Input: part model. Units: mm. Frame: model coordinates. Face numbers are marked on the shaded views. A direction names the side the tool comes from. Give positions to 0.01 mm unless a question says otherwise; leave off trailing zeros. Order: outer loops, then holes, each group sorted by start corner. A loop starts at its lowest first (then second) coordinate and runs counter-clockwise, first axis right, second up. Notation, with made-up numbers: (84.25, 43) - (95.25, 43) arc R12 cw to (95.25, 53) - close; hole circle Ø10 at (-8.75, 35). An arc over 180 degrees is marked (long way). Use a Markdown table: item, result.
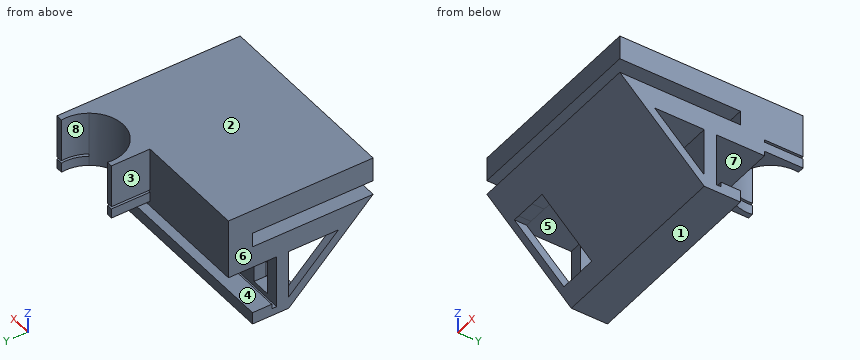
Autodesk Inventor part; units mm, degrees
ref_plane "YZ Plane" through (0, 0, 0) normal (1, 0, 0) x (0, 1, 0)
ref_plane "XZ Plane" through (0, 0, 0) normal (0, 1, 0) x (-1, 0, 0)
ref_plane "XY Plane" through (0, 0, 0) normal (0, 0, 1) x (1, 0, 0)
sketch "Base" plane through (0, 0, 0) normal (1, 0, 0) x (0, 1, 0)
  line L0 (0, 0) -> (0, 6)
  line L1 (0, 6) -> (-50, 6)
  line L2 (-50, 6) -> (-50, 16)
  line L3 (-50, 16) -> (10, 16)
  line L4 (10, -9) -> (-10, -9)
  line L5 (-10, -9) -> (-10, -29)
  line L6 (-10, -29) -> (0, -29)
  line L7 (0, -29) -> (0, -34)
  line L8 (0, -34) -> (-15, -34)
  line L9 (-15, -34) -> (-50, 0)
  line L10 (-50, 0) -> (0, 0)
  line L11 (10, 16) -> (10, -9)
  dimension "d0" = 6
  dimension "d1" = 50
  dimension "d2" = 10
  dimension "d3" = 60
  dimension "d4" = 25
  dimension "d5" = 20
  dimension "d6" = 20
  dimension "d7" = 10
  dimension "d8" = 5
  dimension "d9" = 15
sketch "Mount" plane through (0, 0, 0) normal (1, 0, 0) x (0, 1, 0)
  line L0 (10, 16) -> (26, 16)
  line L1 (26, 16) -> (26, -7)
  line L2 (26, -7) -> (10, -7)
  line L3 (10, -7) -> (10, 16)
  point P0 (0, 0)
  dimension "d13" = 16
  dimension "d14" = 23
extrude "Extrusion1" add sketch "Base" along normal blind 90
extrude "Extrusion2" add sketch "Mount" along normal blind 90
sketch "Sketch4" plane through (0, 10, -7) normal (0, 0, -1) x (-1, 0, 0)
  line L0 (0, 0) -> (0, 16)
  line L1 (0, 16) -> (-90, 16)
  line L2 (-90, 0) -> (-90, 16)
  line L3 (0, 0) -> (-90, 0)
  line L4 (-90, 17.3769) -> (-85, 17.3769)
  line L5 (-85, 17.3769) -> (-85, 0)
  line L6 (0, 0) -> (-90, 0)
  line L7 (-85, 0) -> (-62.2, 0)
  line L8 (-62.2, 0) -> (-62.2, 17.3769)
  line L9 (-62.2, 17.3769) -> (-57.2, 17.3769)
  line L10 (-57.2, 17.3769) -> (-57.2, 0)
  line L11 (-90, 17.3769) -> (-90, 25.7938)
  line L12 (-90, 25.7938) -> (16.0885, 26.6461)
  line L13 (16.0885, 26.6461) -> (17.0474, 0)
  line L14 (17.0474, 0) -> (-57.2, 0)
  point P0 (0, -10)
  dimension "d19" = 5
  dimension "d20" = 22.8
  dimension "d21" = 5
extrude "Extrusion3" cut sketch "Sketch4" against normal blind 90 contours L3 L10 L1 L0 | L0 L1 L10 L9 L8 L5 L4 L11 L12 L13 L14 | L3 L5 L1 L8
sketch "Sketch7" plane through (90, 0, 0) normal (1, 0, 0) x (0, 0, -1)
  line L0 (29, 0) -> (29, -10)
  line L1 (29, -10) -> (9, -10)
  line L2 (9, -10) -> (9, 10)
  line L3 (9, 10) -> (7, 10)
  line L4 (7, 10) -> (7, 26)
  line L5 (7, 26) -> (-16, 26)
  line L6 (-16, 26) -> (-16, -50)
  line L7 (-16, -50) -> (-6, -50)
  line L8 (-6, -50) -> (-6, 0)
  line L9 (-6, 0) -> (0, 0)
  line L10 (0, 0) -> (0, -50)
  line L11 (0, -50) -> (34, -15)
  line L12 (34, -15) -> (34, 0)
  line L13 (34, 0) -> (29, 0)
  line L14 (9, -15) -> (29, -15)
  line L15 (29, -15) -> (9, -35.6361)
  line L16 (9, -35.6361) -> (9, -15)
extrude "Extrusion5" cut sketch "Sketch7" against normal blind 90 contours L14 L15 L16
sketch "Sketch8" plane through (90, 0, 0) normal (1, 0, 0) x (0, 0, -1)
  line L0 (29, -15) -> (9, -35.6361)
  line L1 (9, -35.6361) -> (9, -15)
  line L2 (9, -15) -> (29, -15)
  line L3 (29, 0) -> (29, -10)
  line L4 (29, -10) -> (9, -10)
  line L5 (9, -10) -> (9, 10)
  line L6 (9, 10) -> (7, 10)
  line L7 (7, 10) -> (7, 26)
  line L8 (7, 26) -> (-16, 26)
  line L9 (-16, 26) -> (-16, -50)
  line L10 (-16, -50) -> (-6, -50)
  line L11 (-6, -50) -> (-6, 0)
  line L12 (-6, 0) -> (0, 0)
  line L13 (0, 0) -> (0, -50)
  line L14 (0, -50) -> (34, -15)
  line L15 (34, -15) -> (34, 0)
  line L16 (34, 0) -> (29, 0)
  line L17 (2, 10) -> (3, 10)
  line L18 (2, 10) -> (2, 28)
  line L19 (2, 28) -> (3, 28)
  line L20 (3, 28) -> (3, 10)
  point P0 (-16, 10)
  dimension "d39" = 18
  dimension "d40" = 1
  dimension "d69" = 18
extrude "Extrusion6" cut sketch "Sketch8" against normal blind 90 contours L20 L17 L18 L8 | L8 L18 L19 L20
sketch "Sketch9" plane through (0, -15, -34) normal (0, 0, -1) x (-1, 0, 0)
  line L0 (0, -35) -> (-90, -35)
  line L1 (0, -35) -> (-10, -35)
  line L2 (-10, -35) -> (-10, 26.7876)
  line L3 (-10, 26.7876) -> (0, 26.7876)
  line L4 (0, 26.7876) -> (0, -35)
  point P0 (0, 15)
  dimension "d44" = 10
extrude "Extrusion7" cut sketch "Sketch9" against normal blind 90
sketch "Sketch10" plane through (90, -10, -9) normal (0, 1, 0) x (1, 0, 0)
  line L0 (-74.3662, 20.0264) -> (-66.3662, 20.0264)
  line L1 (-66.3662, 20.0264) -> (-66.3662, 0.0264)
  line L2 (-66.3662, 0.0264) -> (-74.3662, 0.0264)
  line L3 (-74.3662, 0.0264) -> (-74.3662, 20.0264)
  point P0 (-90, -9)
  dimension "d47" = 8
  dimension "d58" = 20
extrude "Extrusion8" cut sketch "Sketch10" against normal blind 90
sketch "Sketch11" plane through (90, -50, 6) normal (0, -1, 0) x (1, 0, 0)
  line L0 (-74.3662, -35.0264) -> (-74.3662, -15.0264)
  line L1 (-74.3662, -15.0264) -> (-66.3662, -15.0264)
  line L2 (-66.3662, -15.0264) -> (-66.3662, -35.0264)
  line L3 (-66.3662, -35.0264) -> (-74.3662, -35.0264)
  line L4 (-80, -6) -> (-80, -40)
  line L5 (-80, -40) -> (0, -40)
  line L6 (0, -6) -> (0, -40)
  line L7 (-80, -6) -> (0, -6)
  line L8 (-60.2122, -34.9767) -> (-76.9534, -34.9767)
  line L9 (-76.9534, -34.9767) -> (-76.9534, -15.0247)
  line L10 (-76.9534, -15.0247) -> (-60.2122, -15.0247)
  line L11 (-60.2122, -15.0247) -> (-60.2122, -34.9767)
  point P0 (-90, -6)
extrude "Extrusion9" cut sketch "Sketch11" against normal blind 35 contours L8 L9 L10 L0 | L2 L10 L11 L8
sketch "Sketch12" plane through (90, 10, -7) normal (0, 0, -1) x (-1, 0, 0)
  line L0 (5, 0) -> (5, 16)
  line L1 (5, 16) -> (0, 16)
  line L2 (0, 0) -> (0, 16)
  line L3 (5, 0) -> (0, 0)
  line L4 (27.8, 16) -> (27.8, 0)
  line L5 (32.8, 0) -> (27.8, 0)
  line L6 (32.8, 0) -> (32.8, 16)
  line L7 (32.8, 16) -> (27.8, 16)
  line L8 (2.5, 7) -> (16.4, 7)
  line L9 (80, 0) -> (0, 0)
  point P0 (90, -10)
  point P1 (30.282, 6.0006)
  dimension "d52" = 27.8
  dimension "d53" = 13.9
  dimension "d70" = 7
sketch "Sketch13" plane through (90, 0, 0) normal (1, 0, 0) x (0, 0, -1)
  line L0 (2, 10) -> (2, 26)
  line L1 (2, 26) -> (-16, 26)
  line L2 (-16, 26) -> (-16, -50)
  line L3 (-16, -50) -> (-6, -50)
  line L4 (-6, -50) -> (-6, 0)
  line L5 (-6, 0) -> (0, 0)
  line L6 (0, 0) -> (0, -50)
  line L7 (0, -50) -> (34, -15)
  line L8 (34, -15) -> (34, 0)
  line L9 (34, 0) -> (29, 0)
  line L10 (29, 0) -> (29, -10)
  line L11 (29, -10) -> (9, -10)
  line L12 (9, -10) -> (9, 10)
  line L13 (9, 10) -> (7, 10)
  line L14 (7, 10) -> (7, 26)
  line L15 (3, 26) -> (3, 10)
  line L16 (3, 10) -> (2, 10)
  line L17 (29, -15) -> (9, -35.6361)
  line L18 (9, -35.6361) -> (9, -15)
  line L19 (9, -15) -> (29, -15)
  line L20 (29, -10) -> (9, -10)
  line L21 (29, -10) -> (31, -10)
  line L22 (31, -10) -> (31, -8)
  line L23 (31, -8) -> (29, -8)
  line L24 (29, 0) -> (29, -10)
  line L25 (29, -10) -> (29, -8)
  line L26 (7, 26) -> (3, 26)
  dimension "d54" = 2
  dimension "d55" = 2
extrude "Extrusion10" cut sketch "Sketch13" against normal through all contours L10 L23 L22 L21
sketch "Sketch15" plane through (90, 10, -7) normal (0, 0, -1) x (-1, 0, 0)
  line L0 (5, 0) -> (5, 16)
  line L1 (5, 16) -> (0, 16)
  line L2 (0, 0) -> (0, 16)
  line L3 (5, 0) -> (0, 0)
  line L4 (27.8, 16) -> (27.8, 0)
  line L5 (32.8, 0) -> (27.8, 0)
  line L6 (32.8, 0) -> (32.8, 16)
  line L7 (32.8, 16) -> (27.8, 16)
  line L8 (80, 0) -> (0, 0)
  circle A0 centre (16.6079, 14) radius 14 construction
  line L9 (27.8, 0) -> (27.8, 16)
  line L10 (27.8, 5.5895) -> (27.8, 16)
  line L11 (27.8, 16) -> (30.4643, 16)
  line L12 (32.8, 16) -> (27.8, 16)
  arc A1 (27.8, 5.5895) -> (30.4643, 16) centre (16.6079, 14) ccw
  line L13 (5, 16) -> (0, 16)
  line L14 (5, 16) -> (5, 0)
  arc A2 (2.7515, 16) -> (5, 6.1733) centre (16.6079, 14) ccw
  line L15 (5, 16) -> (2.7515, 16)
  line L16 (5, 6.1733) -> (5, 16)
  point P0 (90, -10)
  point P1 (27.8, 5.5895)
  point P2 (30.4643, 16)
  point P3 (2.7515, 16)
  point P4 (5, 6.1733)
  dimension "d63" = 14
  dimension "d64" = 28
extrude "Extrusion12" cut sketch "Sketch15" against normal up to surface (23 mm away) contours A2 L1 L0 | L4 L7 A1
sketch "Sketch16" plane through (90, 10, -7) normal (0, 0, -1) x (-1, 0, 0)
  circle A0 centre (16.6079, 14) radius 14 construction
  line L0 (5, 0) -> (5, 6.1733)
  line L1 (5, 6.1733) -> (5, 0)
  line L2 (5, 0) -> (27.7766, 0)
  line L3 (80, 0) -> (0, 0)
  line L4 (27.8, 0) -> (27.8, 5.5895)
  line L5 (27.8, 5.5895) -> (27.8, 0)
  line L6 (5, 0) -> (0, 0)
  line L7 (27.8, 0) -> (5, 0)
  line L8 (5, 0) -> (5, 6.1733)
  line L9 (32.8, 0) -> (27.8, 0)
  line L10 (5, 0) -> (27.8, 0)
  arc A1 (5, 6.1733) -> (27.8, 5.5895) centre (16.6079, 14) ccw
  point P0 (90, -10)
  point P1 (16.6079, 0)
extrude "Extrusion13" add sketch "Sketch16" against normal up to surface (23 mm away)
properties part number "Base Part"
1. Section query D-D (x = 83). Return loops of the section in (y, z), then the cut area to 3 significant figures.
Response:
| item | result |
|---|---|
| outline | (-50, 0) - (-15, -34) - (0, -34) - (0, -29) - (-8, -29) - (-8, -31) - (-10, -31) - (-10, -9) - (10, -9) - (10, -7) - (13.82, -7) - (13.82, 16) - (-50, 16) - (-50, 6) - (0, 6) - (0, 0) - close; hole (-35.64, -9) - (-15, -29) - (-15, -9) - close |
| area | 1,530 mm^2 |
2. Section query B-B (z = -17.5). Return loops of the section in (x, y), then the cut area to 3 significant figures.
Response:
| item | result |
|---|---|
| outline | (10, -31.99) - (13.05, -31.99) - (13.05, -26.87) - (10, -26.87) - close; (10, -15) - (15.63, -15) - (15.63, -10) - (10, -10) - close; (23.63, -15) - (90, -15) - (90, -10) - (23.63, -10) - close; (29.79, -31.99) - (90, -31.99) - (90, -26.87) - (29.79, -26.87) - close |
| area | 684 mm^2 |
3. Section query C-C (y = -29). Return loops of the section in (x, z).
Response:
| item | result |
|---|---|
| outline | (10, -20.4) - (13.05, -20.4) - (13.05, -15.43) - (10, -15.43) - close; (10, -9) - (90, -9) - (90, 0) - (10, 0) - close; (10, 6) - (90, 6) - (90, 16) - (10, 16) - close; (29.79, -20.4) - (90, -20.4) - (90, -15.43) - (29.79, -15.43) - close |
4. Set-up query: the marked faces 1, 2, 3, 4 and 5. Return all of +Z, -Z, +X, -X, +Y, -Y with unobstructed straight access to the full face (end or side cutting, diameter ignored); none if empty.
Response:
| item | result |
|---|---|
| face 1 | -Z, +X, -X, +Y, -Y |
| face 2 | +Z, +X, -X, +Y, -Y |
| face 3 | +Z, -Z, -X, +Y |
| face 4 | +X, -X, +Y |
| face 5 | +X, -X |
5. Section query A-A (y = -9). Return loops of the section in (x, z).
Response:
| item | result |
|---|---|
| outline | (10, -34) - (90, -34) - (90, -31) - (10, -31) - close; (10, -9) - (90, -9) - (90, 0) - (10, 0) - close; (10, 6) - (90, 6) - (90, 16) - (10, 16) - close |
6. Pin query (flat end, axial travel): pin 1 (10 mm diameter, centred on x = 45.5, z = -5, fed in from +Y); pin 2 (13 mm diameter, centred on x = 65, y = 20.5, fed in from -Z); pin 3 (8 mm diameter, centred on y = 22, z = 5.5, fed in from -X). Return the tip coordinate at first contact, or that it passes through.
Response:
| item | result |
|---|---|
| pin 1 | stops at y = 10 |
| pin 2 | stops at z = -7 |
| pin 3 | stops at x = 57.2 |
7. Material intervals for line 1 along Z through (x, y) = (21, -12); line 2 along Z through (x, y) = (34.5, -19); line 3 along X through (y, z) = (-13, -19.5), sorted ascending.
Response:
| item | result |
|---|---|
| line 1 | z = -34 to -29.03, -9.03 to 0, 6 to 16 |
| line 2 | z = -30.11 to -25.12, -9 to 0, 6 to 16 |
| line 3 | x = 10 to 15.63, 23.63 to 90 |
8. Mould query, pull axis X, two halves, no side actions, for the marked faces 6, 7 and 8. Classes: pulls with the +X half, pulls with the -X half, needs draft (parallel to the pull), parting line crosses it, or undercut.
Response:
| item | result |
|---|---|
| face 6 | pulls with the -X half |
| face 7 | needs draft |
| face 8 | undercut |
